The listing builds one solid part. Answer for the finished solid, in the listing's coordinates (mm). A direction names the side the tool comes from. Coordinates: 2 decimals unless noted, no trailing zeros. Write each loop counter-clockwise with the first axis right and the second up, starting at its lowest first coordinate (ties: lowest second). Pieces come first, ordered by that corner, then holes.
from build123d import *

# Parameters (mm, degrees)
ESQUISSE1_R                  = 60
BOSS_EXTRU_1_DEPTH           = 25
ESQUISSE2_R                  = 18
ENL_V_MAT_EXTRU_1_DEPTH      = 3
ENL_V_MAT_EXTRU_2_DEPTH      = 88.658428003
ENL_V_MAT_EXTRU_2_DEPTH_BACK = 88.658428003
ESQUISSE3_R                  = 5
ESQUISSE4_W                  = 45
ESQUISSE4_H                  = 16
ESQUISSE4_W_2                = 16
ESQUISSE4_H_2                = 45
ENL_V_MAT_EXTRU_3_DEPTH      = 16


with BuildPart() as part:
    # Esquisse1 → Boss.-Extru.1 (new body)
    with BuildSketch(Plane.XY):
        Circle(ESQUISSE1_R)
    extrude(amount=BOSS_EXTRU_1_DEPTH)

    # Esquisse2 → Enlèv. mat.-Extru.1 (cut)
    with BuildSketch(Plane.XY.offset(25)):
        Circle(ESQUISSE2_R)
    extrude(amount=-ENL_V_MAT_EXTRU_1_DEPTH, mode=Mode.SUBTRACT)

    # Esquisse3 → Enlèv. mat.-Extru.2 (cut, two sides: drawn at the far end of the back side and taken through both)
    with BuildSketch(Plane.XY.offset(22).offset(-ENL_V_MAT_EXTRU_2_DEPTH_BACK)):
        Circle(ESQUISSE3_R)
    extrude(amount=ENL_V_MAT_EXTRU_2_DEPTH + ENL_V_MAT_EXTRU_2_DEPTH_BACK, mode=Mode.SUBTRACT)

    # Esquisse4 → Enlèv. mat.-Extru.3 (cut)
    with BuildSketch(Plane(origin=(0, 0, 0), x_dir=(-1, 0, 0), z_dir=(0, 0, -1))):
        with Locations((37.5, 0)):
            Rectangle(ESQUISSE4_W, ESQUISSE4_H)
        with Locations((0, -37.5)):
            Rectangle(ESQUISSE4_W_2, ESQUISSE4_H_2)
        with Locations((-37.5, 0)):
            Rectangle(ESQUISSE4_W, ESQUISSE4_H)
        with Locations((0, 37.5)):
            Rectangle(ESQUISSE4_W_2, ESQUISSE4_H_2)
    extrude(amount=-ENL_V_MAT_EXTRU_3_DEPTH, mode=Mode.SUBTRACT)


solid = part.part
1. Section B-B on z = 7.75 is taken. Give the vertices of the cut face in (x, y).
Results found:
outline: (-59.46, -8) arc R60 ccw to (-8, -59.46) - (-8, -15) - (8, -15) - (8, -59.46) arc R60 ccw to (59.46, -8) - (15, -8) - (15, 8) - (59.46, 8) arc R60 ccw to (8, 59.46) - (8, 15) - (-8, 15) - (-8, 59.46) arc R60 ccw to (-59.46, 8) - (-15, 8) - (-15, -8) - close; hole circle Ø10 at (0, 0)
2. Find the intervals of material crossed by L1, parallel to X at y = 0, z = 12.5; L2, parallel to Y at x = -0.5, z = 4; L3, parallel to Z at x = 8.5, y = -4, in increasing order.
Results found:
L1: x = -15 to -5, 5 to 15
L2: y = -15 to -4.97, 4.97 to 15
L3: z = 0 to 22
3. Section D-D on x = -48 is taken. Give the vertices of the cut face in (y, z), then the cut area to 3 significant figures.
Results found:
outline: (-36, 0) - (-8, 0) - (-8, 16) - (8, 16) - (8, 0) - (36, 0) - (36, 25) - (-36, 25) - close
area: 1,540 mm2
4. A tool of negligible diameter and unlimited length cuts with its end or side. For faces 4 (the flat face through (0, -37, 16)), 5 (the flat face through (38, 0, 16)), 6 (the flat face through (0, 38, 16)), 7 (the flat face through (-15, 0, 8)), from which of +Z, -Z, +X, -X, +Y, -Y can it reach the whole face along a straight path? Write none if from no direction.
Results found:
face 4: -Z, -Y
face 5: -Z, +X
face 6: -Z, +Y
face 7: -Z, -X
5. Flat-ended cylindrical pins translate along their axes: P1, Ø13, axis at x = 0, y = 0, coming from the +Z side; P2, Ø2, axis at x = 36.5, z = 8.5, coming from the -Y side; P3, Ø13, axis at y = -0.5, z = 8.5, coming from the +X side. Find the tip coordinate at first contact, or state that the pin passes through.
Results found:
P1: stops at z = 22
P2: stops at y = -48.37
P3: stops at x = 15
6. For a pull along Y with two mould halves and no side action, classify faces 1 (the flat face through (12, 14, 25)), 2 (the cylindrical face through (27.69, -53.23, 12.32)), 3 (the flat face through (15, 0, 8)) as pulls with the +Y half, pulls with the -Y half, needs draft (parallel to the pull), parting line crosses it, or undercut.
Results found:
face 1: needs draft
face 2: parting line crosses it
face 3: undercut
7. Section A-A on y = 0 is taken. Give the vertices of the cut face in (x, z).
Results found:
outline: (-60, 16) - (-15, 16) - (-15, 0) - (-5, 0) - (-5, 22) - (-18, 22) - (-18, 25) - (-60, 25) - close; (5, 0) - (15, 0) - (15, 16) - (60, 16) - (60, 25) - (18, 25) - (18, 22) - (5, 22) - close
